Can you work these out from the model? Positions are in its coordinate system, mm. A direction names the side the tool comes from. Coordinates: 2 decimals unless noted, no trailing zeros. Order: outer loops, then holes, each group sorted by start corner. A loop starts at its lowest first (then second) coordinate and runs counter-clockwise, first axis right, second up. Notation, with made-up numbers: M -21,1 L 6,1 A28 cw 6,38 Z; hole C 36.5,56.25 d11. An arc over 180 degrees is marked long. Answer as a JSON object with one key per item and string values.
from build123d import *

# Parameters (mm, degrees)
PAD_DEPTH       = 30
SKETCH001_R     = 2.5
POCKET_DEPTH    = 3.001
SKETCH002_R     = 2.5
POCKET001_DEPTH = 5
FILLET_R        = 2.5
CHAMFER_SIZE    = 1


with BuildPart() as part:
    # Sketch → Pad (new body)
    with BuildSketch(Plane.XY):
        Polygon((-3, 19), (0, 19), (0, 3), (25, 3), (25, 0), (0, 0), (-3, 0), align=None)
    extrude(amount=PAD_DEPTH)

    # Sketch001 (on Face2 of Pad) → Pocket (cut, through all)
    with BuildSketch(Plane.YZ):
        with Locations((11, 8)):
            Circle(SKETCH001_R)
    extrude(amount=-POCKET_DEPTH, mode=Mode.SUBTRACT)

    # Sketch002 (on Face8 of Pocket) → Pocket001 (cut)
    with BuildSketch(Plane(origin=(0, 3, 0), x_dir=(-1, 0, 0), z_dir=(0, 1, 0))):
        with Locations((-12.5, 20)):
            Circle(SKETCH002_R)
    extrude(amount=-POCKET001_DEPTH, mode=Mode.SUBTRACT)

    # Fillet
    fillet_edges = [part.edges().sort_by_distance(p)[0] for p in [
        (25, 1.5, 0),
        (25, 1.5, 30),
        (-1.5, 19, 30),
        (-1.5, 19, 0),
    ]]
    fillet(fillet_edges, radius=FILLET_R)

    # Chamfer
    chamfer_edges = [part.edges().sort_by_distance(p)[0] for p in [
        (-3, 8.5, 8),
    ]]
    chamfer(chamfer_edges, length=CHAMFER_SIZE)


solid = part.part
Item 1: I want a section at A-A, the plane x = 12.5. Write out the boundary of the cut face in (y, z).
Answers follow:
{"outline": "M 0,0 L 3,0 L 3,17.5 L 0,17.5 Z; M 0,22.5 L 3,22.5 L 3,30 L 0,30 Z"}
Item 2: Which directions (+Z, -Z, +X, -X, +Y, -Y) give clear straight access to the entire face, cutting with the end or side of a thin tool? Please do faces 4 (the flat face through (0, 11, 15)), 5 (the cylindrical face through (-0.99, 10.46, 5.56)).
Answers follow:
{"face 4": "+Z, -Z, +X, +Y", "face 5": "+X, -X"}
Item 3: I'm going to push flat-ended pins straight in: pin 1 (5 mm diameter, centred on y = 7.5, z = 16, fed in from +X); pin 2 (1.5 mm diameter, centred on x = 19.5, z = 15, fed in from +Y). Where does each tip first touch, or does it pass through?
Answers follow:
{"pin 1": "stops at x = 0", "pin 2": "stops at y = 3"}
Item 4: I want a section at D-D, the plane z = 8. Write out the boundary of the cut face in (x, y).
Answers follow:
{"outline": "M -3,0 L 25,0 L 25,3 L 0,3 L 0,8.5 L -2,8.5 L -3,7.5 Z; M -3,14.5 L -2,13.5 L 0,13.5 L 0,19 L -3,19 Z"}
Item 5: Please list where these lines run through material, in increasing order: line 1 (Z direction, x = 12.5, y = 2); line 2 (X direction, y = 15, z = 28); line 3 (Y direction, x = 1.25, z = 24.75).
Answers follow:
{"line 1": "z = 0 to 17.5, 22.5 to 30", "line 2": "x = -3 to 0", "line 3": "y = 0 to 3"}
Item 6: I want a section at B-B, the plane z = 20. Write out the boundary of the cut face in (x, y).
Answers follow:
{"outline": "M -3,0 L 10,0 L 10,3 L 0,3 L 0,19 L -3,19 Z; M 15,0 L 25,0 L 25,3 L 15,3 Z"}
Item 7: I want a section at C-C, the plane y = 11. Write out the boundary of the cut face in (x, z), plus the area to 3 significant figures.
Answers follow:
{"outline": "M -3,0 L 0,0 L 0,5.5 L -2,5.5 L -3,4.5 Z; M -3,11.5 L -2,10.5 L 0,10.5 L 0,30 L -3,30 Z", "area": "74.0 mm^2"}
Item 8: If we mould it in two halves opening along X, with no side actions, what happens to faces 1 (the cylindrical face through (24.248, 1.479, 29.287)), 2 (the cylindrical face through (-1.479, 18.287, 0.752)), 3 (the cylindrical face through (12.83, 1.52, 22.48))? For each: pulls with the +X half, pulls with the -X half, needs draft (parallel to the pull), parting line crosses it, or undercut.
Answers follow:
{"face 1": "pulls with the +X half", "face 2": "needs draft", "face 3": "undercut"}
